Geometry check sheet. Reference: the model listing, model coordinates, mm. Face numbers are marked on the shaded views. A direction names the side the tool comes from. Give positions to 0.01 mm unless a question says otherwise; leave off trailing zeros. Order: outer loops, then holes, each group sorted by start corner. A loop starts at its lowest first (then second) coordinate and runs counter-clockwise, first axis right, second up. Notation, with made-up numbers: M 7.5,77 L 59.5,77 A25 cw 59.5,94 Z; hole C -28,46.25 d7. An arc over 180 degrees is marked long. Put each result on its own line as item: value. Start each with the question number.
Q1. Section check C-C on y = 3.25. Record the cut outline in (x, z).
Q2. Section check B-B on z = 6. Record the cut outline in (x, y).
Q3. Access from +Z, -Z, +X, -X, +Y, -Y to the whole of each face (thin tool, end or side, straight path). Record for the marked faces 1 and 2.
Q4. Section check D-D on x = -4.25. Record the cut outline in (y, z), then the cut area to 3 significant figures.
Q5. Section check A-A on x = 0. Record the cut outline in (y, z), then the cut area to 3 significant figures.
Q6. Go/stop test with flat-tipped pins: pin 1 (8 mm diameter, centred on x = -3, y = 2, fed in from +Z); pin 2 (2 mm diameter, centred on y = -5.5, z = 7, fed in from +X); pin 3 (1 mm diameter, centred on x = 6.5, z = 2.5, fed in from +Y) (3 decimals). Record where each tip stops, or that it passes through.
Q7. Material ranges on L1, parallel to Y at x = 0, z = 1.5; L2, parallel to Y at x = -5, z = 4.5; L3, parallel to X at y = 4.75, z = 7, recorded low to high.
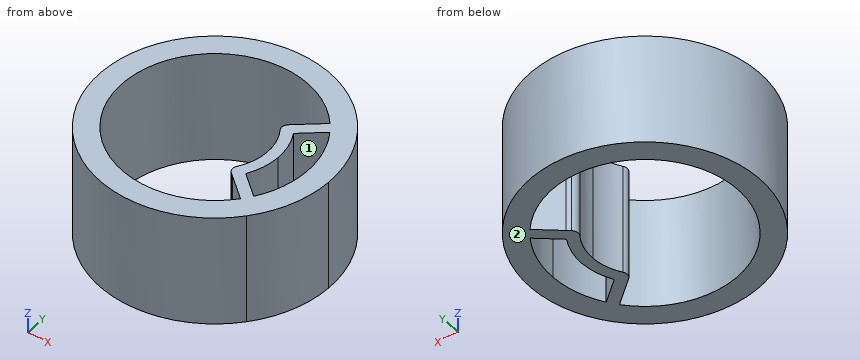
```python
from build123d import *

# Parameters (mm, degrees)
F1_DEPTH = 8
F2_R     = 0.5


with BuildPart() as f1:
    # F0 (on Top) → F1 (new body)
    with BuildSketch(Plane.XY):
        with BuildLine():
            ThreePointArc((5.1324977689, -4.3066769849), (-6.7, 0), (5.1324977689, 4.3066769849))
            Line((5.1324977689, 4.3066769849), (6.3581688779, 5.3351371604))
            ThreePointArc((6.3581688779, 5.3351371604), (-8.3, 0), (6.3581688779, -5.3351371604))
            Line((6.3581688779, -5.3351371604), (5.1324977689, -4.3066769849))
        make_face()
        with BuildLine():
            Line((6.3581688779, 5.3351371604), (5.1324977689, 4.3066769849))
            ThreePointArc((5.1324977689, 4.3066769849), (5.3808860494, 3.9920001658), (5.6100093148, 3.6630309155))
            ThreePointArc((5.6100093148, 3.6630309155), (6.4217233828, 1.9108816801), (6.7, 0))
            ThreePointArc((6.7, 0), (6.4217233828, -1.9108816801), (5.6100093148, -3.6630309155))
            ThreePointArc((5.6100093148, -3.6630309155), (5.3808860494, -3.9920001658), (5.1324977689, -4.3066769849))
            Line((5.1324977689, -4.3066769849), (6.3581688779, -5.3351371604))
            ThreePointArc((6.3581688779, -5.3351371604), (7.7994487525, -2.8387671896), (8.3, 0))
            ThreePointArc((8.3, 0), (7.7994487525, 2.8387671896), (6.3581688779, 5.3351371604))
        make_face()
        with BuildLine():
            Line((5.1324977689, 4.3066769849), (3.5238044383, 2.9568230046))
            ThreePointArc((3.5238044383, 2.9568230046), (3.7684541862, 2.6379448528), (3.9843353171, 2.2989284636))
            Line((3.9843353171, 2.2989284636), (5.6100093148, 3.6630309155))
            ThreePointArc((5.6100093148, 3.6630309155), (5.3808860494, 3.9920001658), (5.1324977689, 4.3066769849))
        make_face()
        with BuildLine():
            ThreePointArc((2.9109688839, 2.4425929168), (3.570831959, 1.2996765446), (3.8, 0))
            ThreePointArc((3.8, 0), (3.570831959, -1.2996765446), (2.9109688839, -2.4425929168))
            Line((2.9109688839, -2.4425929168), (3.5238044383, -2.9568230046))
            ThreePointArc((3.5238044383, -2.9568230046), (3.7684541862, -2.6379448528), (3.9843353171, -2.2989284636))
            ThreePointArc((3.9843353171, -2.2989284636), (4.4434188672, -1.1899700713), (4.6, 0))
            ThreePointArc((4.6, 0), (4.4434188672, 1.1899700713), (3.9843353171, 2.2989284636))
            ThreePointArc((3.9843353171, 2.2989284636), (3.7684541862, 2.6379448528), (3.5238044383, 2.9568230046))
            Line((3.5238044383, 2.9568230046), (2.9109688839, 2.4425929168))
        make_face()
        with BuildLine():
            ThreePointArc((3.9843353171, -2.2989284636), (3.7684541862, -2.6379448528), (3.5238044383, -2.9568230046))
            Line((3.5238044383, -2.9568230046), (5.1324977689, -4.3066769849))
            ThreePointArc((5.1324977689, -4.3066769849), (5.3808860494, -3.9920001658), (5.6100093148, -3.6630309155))
            Line((5.6100093148, -3.6630309155), (3.9843353171, -2.2989284636))
        make_face()
    extrude(amount=F1_DEPTH)

    # F2
    f2_edges = [f1.edges().sort_by_distance(p)[0] for p in [
        (2.910969, 2.442593, 4),
        (2.910969, -2.442593, 4),
    ]]
    fillet(f2_edges, radius=F2_R)


solid = f1.part
```
Results found:
1. outline: M -7.64,0 L -5.86,0 L -5.86,8 L -7.64,8 Z; M 3.87,0 L 5.12,0 L 5.12,8 L 3.87,8 Z; M 5.86,0 L 7.64,0 L 7.64,8 L 5.86,8 Z
2. outline: C 0,0 d16.6; hole M 3.18,-2.09 A3.8 ccw 3.18,2.09 A0.5 cw 3.27,2.75 L 5.13,4.31 A6.7 ccw long 5.13,-4.31 L 3.27,-2.75 A0.5 cw Z; hole M 3.98,-2.3 L 5.61,-3.66 A6.7 ccw 5.61,3.66 L 3.98,2.3 A4.6 cw Z
3. face 1: +Z, -Z
3. face 2: -Z, +X, -X, +Y, -Y
4. outline: M -7.13,0 L -5.18,0 L -5.18,8 L -7.13,8 Z; M 5.18,0 L 7.13,0 L 7.13,8 L 5.18,8 Z
4. area: 31.2 mm^2
5. outline: M -8.3,0 L -6.7,0 L -6.7,8 L -8.3,8 Z; M 6.7,0 L 8.3,0 L 8.3,8 L 6.7,8 Z
5. area: 25.6 mm^2
6. pin 1: stops at z = 8
6. pin 2: stops at x = 6.97
6. pin 3: stops at y = 5.735
7. L1: y = -8.3 to -6.7, 6.7 to 8.3
7. L2: y = -6.62 to -4.46, 4.46 to 6.62
7. L3: x = -6.81 to -4.73, 4.73 to 6.81
